Read the model definition and answer for the solid it produces. Units are mm, in the model's axes. Face numbers are marked on the shaded views. A direction names the side the tool comes from. Give positions to 0.01 mm unless a question says otherwise; leave off trailing zeros. Order: outer loops, then holes, each group sorted by start corner. A loop starts at its lowest first (then second) coordinate and runs counter-clockwise, first axis right, second up.
```python
from build123d import *

# Parameters (mm, degrees)
BOX007_W     = 42
BOX007_H     = 52
BOX007_DEPTH = 9.5
BOX008_W     = 5
BOX008_H     = 10
BOX008_DEPTH = 9.5


with BuildPart() as cube006:
    # Box007 → Box007 (new body)
    with BuildSketch(Plane.XY):
        with Locations((21, 26)):
            Rectangle(BOX007_W, BOX007_H)
    extrude(amount=BOX007_DEPTH)


with BuildPart() as usb_fusion:
    # Box008 → Box008 (new body)
    with BuildSketch(Plane(origin=(42, 21, 0), x_dir=(1, 0, 0), z_dir=(0, 0, 1))):
        with Locations((2.5, 5)):
            Rectangle(BOX008_W, BOX008_H)
    extrude(amount=BOX008_DEPTH)

    # Fusion001: union Cube006
    add(cube006.part)


solid = usb_fusion.part
```
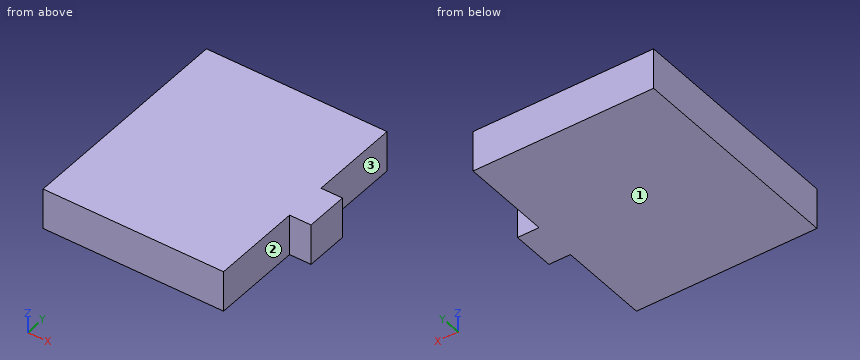
1) The part is cut by section B-B on x = 43.5. Determine the outline of the cut face in (y, z), and give its area (3 significant figures).
Final values:
outline: (21, 0) - (31, 0) - (31, 9.5) - (21, 9.5) - close
area: 95.0 mm2
2) The part is cut by section C-C on y = 34. Determine the outline of the cut face in (x, z).
Final values:
outline: (0, 0) - (42, 0) - (42, 9.5) - (0, 9.5) - close
3) The part is cut by section A-A on z = 6. Determine the outline of the cut face in (x, y), and give its area (3 significant figures).
Final values:
outline: (0, 0) - (42, 0) - (42, 21) - (47, 21) - (47, 31) - (42, 31) - (42, 52) - (0, 52) - close
area: 2,230 mm2
4) Given pin 1 (1.5 mm diameter, centred on x = 45.5, z = 4.5, fed in from +Y); pin 2 (2 mm diameter, centred on x = 20, z = 1.5, fed in from -Y); pin 3 (1.5 mm diameter, centred on x = 44, z = 3.5, fed in from -Y); pin 4 (3 mm diameter, centred on y = 15.5, z = 3, fed in from +X), each flat-ended and moving along its own axis, determine where each tip first touches the part or whether it passes through.
Final values:
pin 1: stops at y = 31
pin 2: stops at y = 0
pin 3: stops at y = 21
pin 4: stops at x = 42
5) Consider L1, parallel to X at y = 37.5, z = 2.75; L2, parallel to Y at x = 44, z = 8.75. Determine where each line is inside the solid, lowest interval first.
Final values:
L1: x = 0 to 42
L2: y = 21 to 31
6) A tool of negligible diameter and unlimited length cuts with its end or side. For the marked faces 1, 2 and 3, from which of +Z, -Z, +X, -X, +Y, -Y can it reach the whole face along a straight path? Write none if from no direction.
Final values:
face 1: -Z, +X, -X, +Y, -Y
face 2: +Z, -Z, +X, -Y
face 3: +Z, -Z, +X, +Y
